from build123d import *

# Parameters (mm, degrees)
BOSS_EXTRUDE1_DEPTH = 5
SKETCH2_R           = 1.95
CUT_EXTRUDE1_DEPTH  = 6


with BuildPart() as part:
    # Sketch1 → Boss-Extrude1 (new body)
    with BuildSketch(Plane(origin=(0, 0, 0), x_dir=(1, 0, 0), z_dir=(0, 1, 0))):
        with BuildLine():
            Line((2, 0), (54, 0))
            ThreePointArc((54, 0), (55.414213562, -0.585786438), (56, -2))
            Line((56, -2), (56, -6))
            ThreePointArc((56, -6), (55.414213562, -7.414213562), (54, -8))
            Line((54, -8), (2, -8))
            ThreePointArc((2, -8), (0.585786438, -7.414213562), (0, -6))
            Line((0, -6), (0, -2))
            ThreePointArc((0, -2), (0.585786438, -0.585786438), (2, 0))
        make_face()
    extrude(amount=BOSS_EXTRUDE1_DEPTH)

    # Sketch2 → Cut-Extrude1 (cut, through all)
    with BuildSketch(Plane(origin=(0, 5, 0), x_dir=(1, 0, 0), z_dir=(0, 1, 0))):
        with Locations((52, -4)):
            Circle(SKETCH2_R)
        with Locations((44, -4)):
            Circle(SKETCH2_R)
        with Locations((-12, -4)):
            Circle(SKETCH2_R)
        with Locations((-4, -4)):
            Circle(SKETCH2_R)
        with Locations((4, -4)):
            Circle(SKETCH2_R)
        with Locations((12, -4)):
            Circle(SKETCH2_R)
        with Locations((20, -4)):
            Circle(SKETCH2_R)
        with Locations((28, -4)):
            Circle(SKETCH2_R)
        with Locations((36, -4)):
            Circle(SKETCH2_R)
    extrude(amount=-CUT_EXTRUDE1_DEPTH, mode=Mode.SUBTRACT)


solid = part.part
Verification items for the finished model (mm, model axes). Coordinates: 2 decimals unless noted, no trailing zeros. Order: outer loops, then holes, each group sorted by start corner. A loop starts at its lowest first (then second) coordinate and runs counter-clockwise, first axis right, second up. Notation, with made-up numbers: M 80.25,22 L 87.25,22 A19 cw 87.25,55 Z; hole C 74,32 d10. An arc over 180 degrees is marked long. Write each question's results on one line, items separated by ' | '.
1) Section check D-D on x = 11.5. Record the cut outline in (y, z), plus the area to 3 significant figures.
Solved:
outline: M 0,0 L 5,0 L 5,2.12 L 0,2.12 Z; M 0,5.88 L 5,5.88 L 5,8 L 0,8 Z | area: 21.2 mm²
2) Section check A-A on z = 4. Give the number of separate pieces and of enclosed holes in the cut face, plus the area to 4 significant figures.
Solved:
separate pieces: 8 | enclosed holes: 0 | area: 143.5 mm²
3) Section check B-B on x = 36. Record the cut outline in (y, z).
Solved:
outline: M 0,0 L 5,0 L 5,2.05 L 0,2.05 Z; M 0,5.95 L 5,5.95 L 5,8 L 0,8 Z
4) Scan lines: line 1 along Z through (x, y) = (20, 3.4); line 2 along Z through (x, y) = (10.5, 1.2); line 3 along X through (y, z) = (1.5, 0.75). Record each from-to range of solid material in increasing order. Write a range as [from, to].
Solved:
line 1: z = [0, 2.05], [5.95, 8] | line 2: z = [0, 2.75], [5.25, 8] | line 3: x = [0.44, 55.56]
5) Gauge pin test, flat end, axial feed: pin 1 Ø1 at (y, z) = (2.5, 1) entering from -X. Record the tip position at first contact, or that the pin passes through.
Solved:
pin 1: stops at x = 0.06
6) Section check C-C on y = 1.65. Record the cut outline in (x, z), plus the area to 3 significant figures.
Solved:
outline: M 0,2 A2 ccw 2,0 L 54,0 A2 ccw 56,2 L 56,6 A2 ccw 54,8 L 2,8 A2 ccw 0,6 Z; hole C 4,4 d3.9; hole C 12,4 d3.9; hole C 20,4 d3.9; hole C 28,4 d3.9; hole C 36,4 d3.9; hole C 44,4 d3.9; hole C 52,4 d3.9 | area: 361 mm²
7) Release check for a two-part mould opening along Z. For faces 1 (the face through (56, 2, 4)), 2 (the face through (28, 2, 8)), 3 (the face through (53.8, 2.54, 4.75)), 4 (the face through (18.052, 2.535, 3.914)) record: pulls with the +Z half, pulls with the -Z half, needs draft (parallel to the pull), parting line crosses it, or undercut.
Solved:
face 1: needs draft | face 2: pulls with the +Z half | face 3: undercut | face 4: undercut
